CAD build for the part. Positions are in the model's coordinates, mm. A direction names the side the tool comes from. Give positions to 0.01 mm unless a question says otherwise; leave off trailing zeros. Loops run counter-clockwise (first coordinate to the right, second up) from the corner with the lowest first, then second, coordinate; pieces in that order, holes last. Notation, with made-up numbers: (46, -28.5) -> (104, -28.5) arc R9 cw to (104, -13.5) -> close; hole circle Ø2 at (18, 82). An arc over 180 degrees is marked (long way). Use one line per item in the form item = value.
Autodesk Inventor part; units mm, degrees
ref_plane "YZ Plane" through (0, 0, 0) normal (1, 0, 0) x (0, 1, 0)
ref_plane "XZ Plane" through (0, 0, 0) normal (0, 1, 0) x (-1, 0, 0)
ref_plane "XY Plane" through (0, 0, 0) normal (0, 0, 1) x (1, 0, 0)
sketch "Sketch1" plane through (0, 0, 0) normal (0, 1, 0) x (-1, 0, 0)
  line L0 (-37, -79.5) -> (37, -79.5)
  line L1 (37, -79.5) -> (37, 79.5)
  line L2 (37, 79.5) -> (-37, 79.5)
  line L3 (-37, 79.5) -> (-37, -79.5)
  line L4 (-37, -79.5) -> (37, 79.5) construction
  line L5 (37, -79.5) -> (-37, 79.5) construction
  point P0 (0, 0)
  dimension "d0" = 74
  dimension "d1" = 159
extrude "Extrusion1" add sketch "Sketch1" along normal blind 3
sketch "Sketch2" plane through (0, 3, 0) normal (0, 1, 0) x (1, 0, 0)
  line L0 (34, 76.5) -> (-34, 76.5)
  line L1 (-34, 76.5) -> (-34, -76.5)
  line L2 (-34, -76.5) -> (34, -76.5)
  line L3 (34, -76.5) -> (34, 76.5)
  line L4 (34, 76.5) -> (-34, -76.5) construction
  line L5 (-34, 76.5) -> (34, -76.5) construction
  line L6 (-37, 79.5) -> (-37, -79.5)
  line L7 (-37, -79.5) -> (37, -79.5)
  line L8 (34, 7) -> (37, 7)
  line L9 (34, -7) -> (37, -7)
  line L10 (37, -79.5) -> (37, 79.5)
  line L11 (34, 32) -> (37, 32)
  line L12 (34, -32) -> (37, -32)
  line L13 (0, 0) -> (0, 8.1012)
  line L14 (-34, 7) -> (-37, 7)
  line L15 (-34, -7) -> (-37, -7)
  line L16 (-34, 32) -> (-37, 32)
  line L17 (-34, -32) -> (-37, -32)
  line L18 (-12.5, -79.5) -> (-12.5, -76.5)
  line L19 (12.5, -76.5) -> (12.5, -79.5)
  line L20 (-34, -32) -> (-34, -7)
  line L21 (-34, 7) -> (-34, -7)
  line L22 (-34, 32) -> (-34, 7)
  line L23 (-37, 7) -> (-37, 32)
  line L24 (-37, -7) -> (-37, -32)
  line L25 (34, -32) -> (34, -7)
  line L26 (37, -7) -> (37, -32)
  line L27 (34, 7) -> (34, 32)
  line L28 (37, 32) -> (37, 7)
  line L29 (12.5, -76.5) -> (-12.5, -76.5)
  line L30 (-12.5, -79.5) -> (12.5, -79.5)
  point P0 (35.5, -7)
  point P1 (34, 0)
  point P2 (35.5, 7)
  point P3 (35.5, 32)
  point P4 (35.5, -32)
  point P5 (0, -76.5)
  point P6 (12.5, -78)
  point P7 (-12.5, -78)
  dimension "d4" = 3
  dimension "d5" = 3
  dimension "d6" = 7
  dimension "d7" = 7
  dimension "d8" = 32
  dimension "d9" = 32
  dimension "d10" = 12.5
  dimension "d11" = 12.5
extrude "Extrusion2" add sketch "Sketch2" along normal blind 108.5 contours L11 L10 L8 L3 | L1 L14 L6 L16 | L9 L10 L12 L3 | L1 L17 L6 L15 | L19 L7 L18 L2
sketch "Sketch3" plane through (-34, 3, 32) normal (1, 0, 0) x (0, 0, -1)
  line L0 (25, 108.5) -> (0, 108.5)
  line L1 (0, 108.5) -> (25, 108.5)
  line L2 (25, 108.5) -> (25, 98.5)
  line L3 (25, 98.5) -> (0, 98.5)
  line L4 (0, 98.5) -> (0, 108.5)
  line L5 (39, 0) -> (39, 108.5)
  line L6 (39, 108.5) -> (64, 108.5)
  line L7 (64, 108.5) -> (64, 98.5)
  line L8 (64, 98.5) -> (39, 98.5)
  line L9 (39, 98.5) -> (39, 108.5)
  point P0 (32, -3)
  dimension "d14" = 25
  dimension "d15" = 10
  dimension "d16" = 25
  dimension "d17" = 10
sketch "Sketch4" plane through (12.5, 3, 76.5) normal (0, 0, -1) x (-1, 0, 0)
  line L0 (0, 108.5) -> (25, 108.5)
  line L1 (0, 108.5) -> (25, 108.5)
  line L2 (25, 108.5) -> (25, 98.5)
  line L3 (25, 98.5) -> (0, 98.5)
  line L4 (0, 98.5) -> (0, 108.5)
  point P0 (12.5, -3)
  dimension "d18" = 25
  dimension "d19" = 10
sketch "Sketch5" plane through (34, 3, 7) normal (-1, 0, 0) x (0, 0, 1)
  line L0 (-14, 108.5) -> (-39, 108.5)
  line L1 (-39, 108.5) -> (-14, 108.5)
  line L2 (-14, 108.5) -> (-14, 98.5)
  line L3 (-14, 98.5) -> (-39, 98.5)
  line L4 (-39, 98.5) -> (-39, 108.5)
  line L5 (0, 108.5) -> (25, 108.5)
  line L6 (25, 108.5) -> (25, 98.5)
  line L7 (25, 98.5) -> (0, 98.5)
  line L8 (0, 98.5) -> (0, 108.5)
  point P0 (-7, -3)
  dimension "d20" = 25
  dimension "d21" = 10
  dimension "d22" = 25
  dimension "d23" = 10
revolve "Revolution1" add sketch "Sketch5" angle 25 about axis through (34, 111.5, 7) along (0, 0, -1)
revolve "Revolution2" add sketch "Sketch4" angle 25 about axis through (12.5, 111.5, 76.5) along (1, 0, 0)
revolve "Revolution3" add sketch "Sketch3" angle 25 about axis through (-34, 111.5, 7) along (0, 0, 1)
sketch "Sketch6" plane through (0, 3, 0) normal (0, 1, 0) x (1, 0, 0)
  line L0 (34, -76.5) -> (-34, -76.5)
  line L1 (-34, -76.5) -> (-34, 76.5)
  line L2 (-34, 76.5) -> (34, 76.5)
  line L3 (34, 76.5) -> (34, -76.5)
  line L4 (12.5, -79.5) -> (37, -79.5)
  line L5 (37, -79.5) -> (37, -32)
  line L6 (-37, -32) -> (-37, -79.5)
  line L7 (37, 79.5) -> (-37, 79.5)
  line L8 (-37, 79.5) -> (-37, -79.5)
  line L9 (37, -79.5) -> (-37, -79.5)
  line L10 (-37, -79.5) -> (-37, 79.5)
  line L11 (-37, 79.5) -> (37, 79.5)
  line L12 (37, 79.5) -> (37, -79.5)
  point P0 (0, 0)
  dimension "d27" = 3
  dimension "d28" = 3
  dimension "d29" = 3
  dimension "d30" = 3
extrude "Extrusion3" add sketch "Sketch6" along normal blind 7
properties part number "battery pack holder"
1. Cut at D-D, the plane z = 28. Write the cut outline in (x, y), then the cut area to 3 significant figures.
Result sheet:
outline = (-37, 0) -> (37, 0) -> (37, 111.5) -> (34, 111.5) -> (29.77, 102.44) arc R10 ccw to (34, 101.5) -> (34, 3) -> (-34, 3) -> (-34, 101.5) arc R10 ccw to (-29.77, 102.44) -> (-34, 111.5) -> (-37, 111.5) -> close
area = 917 mm^2
2. Cut at B-B, the plane z = 67.5. Write the cut outline in (x, y).
Result sheet:
outline = (-37, 0) -> (37, 0) -> (37, 10) -> (34, 10) -> (34, 3) -> (-34, 3) -> (-34, 10) -> (-37, 10) -> close
3. Mould opens along Z. For faces 1 (the flat face through (-35, 60, 7)), 2 (the flat face through (-35, 60, 32)), 3 (the flat face through (31.9, 107, -19.7)) say: pulls with the +Z half, pulls with the -Z half, needs draft (parallel to the pull), parting line crosses it, or undercut.
Result sheet:
face_1 = undercut
face_2 = pulls with the +Z half
face_3 = needs draft
4. Cut at A-A, the plane y = 46.5. Write the cut outline in (x, z), then the cut area to 3 significant figures.
Result sheet:
outline = (-37, -32) -> (-34, -32) -> (-34, -7) -> (-37, -7) -> close; (-37, 7) -> (-34, 7) -> (-34, 32) -> (-37, 32) -> close; (-12.5, 76.5) -> (12.5, 76.5) -> (12.5, 79.5) -> (-12.5, 79.5) -> close; (34, -32) -> (37, -32) -> (37, -7) -> (34, -7) -> close; (34, 7) -> (37, 7) -> (37, 32) -> (34, 32) -> close
area = 375 mm^2
5. Tool access for faces 4 (the flat face through (35, 60, -32)), 5 (the flat face through (35, 60, -7)), 6 (the cylindrical face through (31.87, 101.73, 19.32)): list every direction of +Z, -Z, +X, -X, +Y, -Y with a clear straight run to the whole face (end or side of a thin tool).
Result sheet:
face_4 = -Z, +X, -X, +Y
face_5 = +X, -X, +Y
face_6 = +Z, -Z
6. Drop flat-ended pins along their axis: P1, Ø6, axis at x = 32, y = 75.5, coming from the -Z side; P2, Ø20.5, axis at x = 5, z = 32.5, coming from the +Y side; P3, Ø0.9, axis at x = -35.5, z = 2.5, coming from the +Y side; P4, Ø1, axis at x = 8.5, z = -13, coming from the -Y side. Give the stop position or say it passes through.
Result sheet:
P1 = -32
P2 = 3
P3 = 10
P4 = 0
7. Drill centre lines: line 1 (X direction, y = 60, z = -13.5); line 2 (Z direction, x = -6, y = 5); line 3 (Y direction, x = -8, z = 14.5). Where is each one in solid material? Low to high.
Result sheet:
line_1 = -37 to -34, 34 to 37
line_2 = -79.5 to -76.5, 76.5 to 79.5
line_3 = 0 to 3
8. Cut at C-C, the plane x = 4. Write the cut outline in (y, z), then the cut area to 3 significant figures.
Result sheet:
outline = (0, -79.5) -> (10, -79.5) -> (10, -76.5) -> (3, -76.5) -> (3, 76.5) -> (101.5, 76.5) arc R10 ccw to (102.44, 72.27) -> (111.5, 76.5) -> (111.5, 79.5) -> (0, 79.5) -> close
area = 845 mm^2
